For this review, take the finished solid that the model builds, in its own axes (mm). Give positions to 0.01 mm unless a question says otherwise; leave off trailing zeros. Write each loop counter-clockwise with the first axis right and the second up, starting at its lowest first coordinate (ties: lowest second). Pieces come first, ordered by that corner, then holes. Notation, with made-up numbers: M -38.5,57.5 L -7.5,57.5 A23 cw -7.5,73.5 Z; hole C 11,-26 d6. An arc over 180 degrees is marked long. Use one line per item in the form item = value. Start each with the question number.
Q1. Clearance check with a flat-ended pin moving along its axis: pin 1 Ø5 at (x, y) = (301.72, -106.68) entering from +Z. State where the tip first meets the part, or that it passes through.
Q2. Consider section B-B on x = 351. Write out the cut boundary in (y, z) (3 decimals).
Q3. Consider section A-A on y = -35.5. Write out the cut boundary in (x, z) (3 decimals), and give its area (3 significant figures).
Q4. For probe 1 along Y at (x, z) = (353.5, 2.95); probe 2 along X at (y, z) = (-54, 0.8); probe 3 along X at (y, z) = (-43.5, 2.25), list the stretches that pass through material, from the lowest coordinate up. Write a range as [from, to].
Q5. Consider section C-C on z = 1.9. Give the number of separate pieces and of enclosed holes in the cut face, and give its area (3 significant figures).
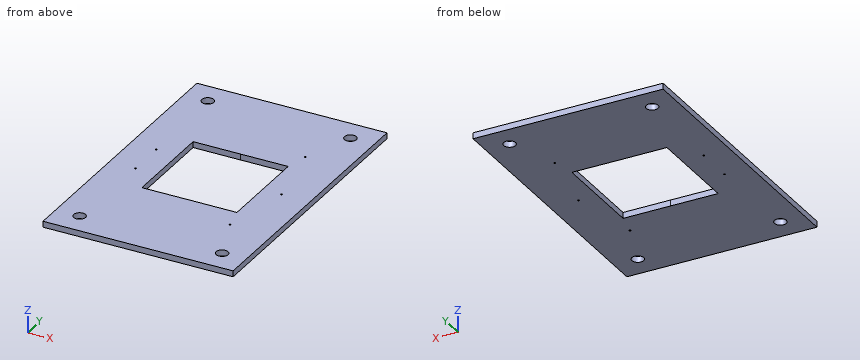
```python
from build123d import *

# Parameters (mm, degrees)
SKETCH2_W           = 101.6
SKETCH2_H           = 152.490905348
SKETCH2_R           = 0.45
BOSS_EXTRUDE1_DEPTH = 3.175
SKETCH3_R           = 3.175
CUT_EXTRUDE1_DEPTH  = 10


with BuildPart() as part:
    # Sketch2 → Boss-Extrude1 (new body)
    with BuildSketch(Plane.XY):
        with Locations((339.823220758, -43.137414152)):
            Rectangle(SKETCH2_W, SKETCH2_H)
        with Locations((302.835020758, -32.804961478)):
            Circle(SKETCH2_R, mode=Mode.SUBTRACT)
        with Locations((367.9685278, -5.825779496)):
            Circle(SKETCH2_R, mode=Mode.SUBTRACT)
        with Locations(Location((302.835020758, -53.469866826, 0), (0, 0, 180))):
            Circle(SKETCH2_R, mode=Mode.SUBTRACT)
        with Locations((375.390273381, -43.137414152)):
            Circle(SKETCH2_R, mode=Mode.SUBTRACT)
        with Locations(Location((367.9685278, -80.449048807, 0), (0, 0, 180))):
            Circle(SKETCH2_R, mode=Mode.SUBTRACT)
        Polygon((365.223220758, -17.737414152), (339.823220758, -17.778276649), (314.423220758, -17.737414152), (314.423220758, -68.537414152), (339.823220758, -68.496551654), (365.223220758, -68.537414152), align=None, mode=Mode.SUBTRACT)
    extrude(amount=BOSS_EXTRUDE1_DEPTH)

    # Sketch3 → Cut-Extrude1 (cut)
    with BuildSketch(Plane.XY.offset(3.175)):
        with Locations((377.923220758, 20.408038522)):
            Circle(SKETCH3_R)
        with Locations(Location((301.723220758, 20.408038522, 0), (0, 0, 180))):
            Circle(SKETCH3_R)
        with Locations((301.723220758, -106.682866826)):
            Circle(SKETCH3_R)
        with Locations(Location((377.923220758, -106.682866826, 0), (0, 0, 180))):
            Circle(SKETCH3_R)
    extrude(amount=-CUT_EXTRUDE1_DEPTH, mode=Mode.SUBTRACT)


solid = part.part
```
Working result:
q1.pin_1 = through
q2.outline = M -119.383,0 L -68.515,0 L -68.515,3.175 L -119.383,3.175 Z; M -17.76,0 L 33.108,0 L 33.108,3.175 L -17.76,3.175 Z
q3.outline = M 289.023,0 L 314.423,0 L 314.423,3.175 L 289.023,3.175 Z; M 365.223,0 L 390.623,0 L 390.623,3.175 L 365.223,3.175 Z
q3.area = 161 mm²
q4.probe_1 = [-119.38, -68.52], [-17.76, 33.11]
q4.probe_2 = [289.02, 314.42], [365.22, 390.62]
q4.probe_3 = [289.02, 314.42], [365.22, 375.12], [375.66, 390.62]
q5.separate_pieces = 1
q5.enclosed_holes = 10
q5.area = 12,800 mm²
